Here's the drawing with two shaded views (mm, measured from the low corner). I have some questions. Round coordinates to 2 decimals unless told otherwise and drop trailing zeros. Write each loop counter-clockwise with the first axis right and the second up, starting at its lowest first coordinate (ties: lowest second). Pieces come first, ordered by that corner, then holes. Notation, with made-up numbers: (60, 51) - (92, 51) arc R9 ccw to (92, 56) - close; hole circle Ø7 at (43, 60). An arc over 180 degrees is marked (long way). Return JSON: item names as keys, results as strings. Group by question number.
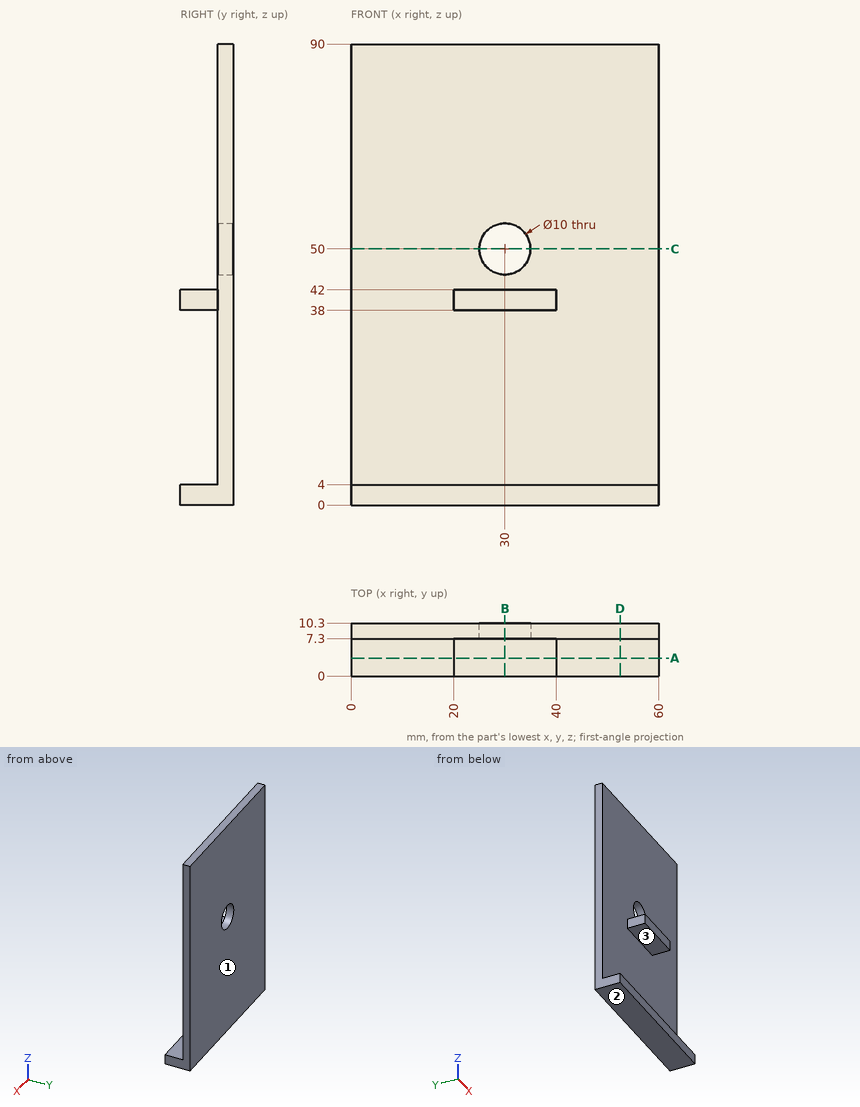
1) Will these pins go through, and if not, where does the flat tip stop? pin 1 Ø1 at (x, y) = (50, 4) entering from +Z; pin 2 Ø1.2 at (y, z) = (4.5, 39.5) entering from +X; pin 3 Ø2 at (x, y) = (29.5, 3) entering from -Z; pin 4 Ø8 at (x, z) = (30, 50) entering from -Y.
2) Imagine slicing it at D-D (x = 52.5). Please give me the cut outline in (y, z), plus the area to 3 significant figures.
3) If we mould it in two halves opening along Z, with no side actions, what happens to the marked faces 1, 2 and 3? For each: released by +Z, released by -Z, zero draft, split by the parting line, or undercut.
4) I need wall thicknesses on line 1 along Z through (x, y) = (23.5, 2); line 2 along Z through (x, y) = (30, 9.45); line 3 along X through (y, z) = (7.95, 50). Which ranges of each line are inside material? Lowest first, please.
5) Imagine slicing it at B-B (x = 30). Please give me the cut outline in (y, z), plus the area to 3 significant figures.
6) Imagine slicing it at C-C (z = 50). Please give me the cut outline in (x, y), plus the area to 3 significant figures.
7) Imagine slicing it at A-A (y = 3.5). Please give me the cut outline in (x, z), plus the area to 3 significant figures.
Results found:
{
 "1": {"pin 1": "stops at z = 4", "pin 2": "stops at x = 40", "pin 3": "stops at z = 0", "pin 4": "passes through"},
 "2": {"outline": "(0, 0) - (10.3, 0) - (10.3, 90) - (7.3, 90) - (7.3, 4) - (0, 4) - close", "area": "299 mm²"},
 "3": {"face 1": "zero draft", "face 2": "released by -Z", "face 3": "undercut"},
 "4": {"line 1": "z = 0 to 4, 38 to 42", "line 2": "z = 0 to 45, 55 to 90", "line 3": "x = 0 to 25, 35 to 60"},
 "5": {"outline": "(0, 0) - (10.3, 0) - (10.3, 45) - (7.3, 45) - (7.3, 42) - (0, 42) - (0, 38) - (7.3, 38) - (7.3, 4) - (0, 4) - close; (7.3, 55) - (10.3, 55) - (10.3, 90) - (7.3, 90) - close", "area": "298 mm²"},
 "6": {"outline": "(0, 7.3) - (25, 7.3) - (25, 10.3) - (0, 10.3) - close; (35, 7.3) - (60, 7.3) - (60, 10.3) - (35, 10.3) - close", "area": "150 mm²"},
 "7": {"outline": "(0, 0) - (60, 0) - (60, 4) - (0, 4) - close; (20, 38) - (40, 38) - (40, 42) - (20, 42) - close", "area": "320 mm²"}
}
